```python
from build123d import *

# Parameters (mm, degrees)
BOSS_EXTRUDE1_DEPTH = 3
CUT_EXTRUDE3_DEPTH  = 4


with BuildPart() as part:
    # Sketch1 → Boss-Extrude1 (new body)
    with BuildSketch(Plane(origin=(0, 0, 0), x_dir=(1, 0, 0), z_dir=(0, 1, 0))):
        Polygon((-6, 15), (-9, 15), (-9, 0), (9, 0), (9, 15), (6, 15), (0, 9), align=None)
    extrude(amount=BOSS_EXTRUDE1_DEPTH)

    # Sketch6 → Cut-Extrude3 (cut, through all)
    with BuildSketch(Plane(origin=(0, 0, 0), x_dir=(1, 0, 0), z_dir=(0, 1, 0))):
        Polygon((-5.9, 3.1), (-5.9, 10.1), (-9.1, 10.1), (-9.1, -0.1), (-2.4, -0.1), (-2.4, 3.1), align=None)
        Polygon((9.1, 10.1), (5.9, 10.1), (5.9, 3.1), (2.4, 3.1), (2.4, -0.1), (9.1, -0.1), align=None)
    extrude(amount=CUT_EXTRUDE3_DEPTH, mode=Mode.SUBTRACT)


solid = part.part
```
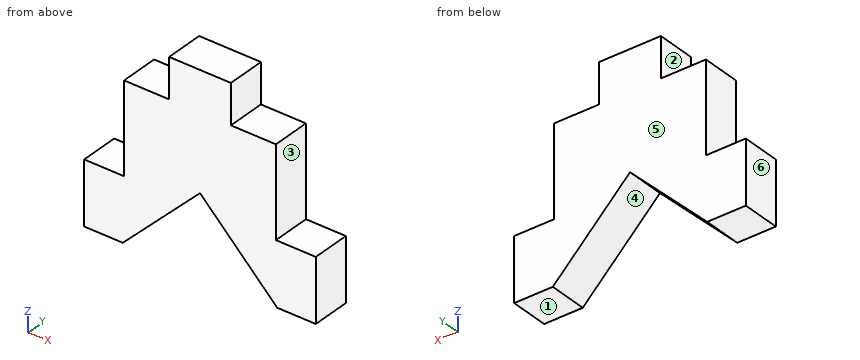
The listing builds one solid part. Answer for the finished solid, in the listing's coordinates (mm). Face numbers are marked on the shaded views. A direction names the side the tool comes from. Coordinates: 2 decimals unless noted, no trailing zeros. Write each loop counter-clockwise with the first axis right and the second up, starting at its lowest first coordinate (ties: lowest second). Pieces come first, ordered by that corner, then holes.
Q1. Given P1, Ø4, axis at x = -6.5, z = -13, coming from the -Y side; P2, Ø0.9, axis at y = 1.5, z = -5, coming from the -X side; P3, Ø0.9, axis at x = -3.5, y = 2, coming from the +Z side; P4, Ø0.9, axis at y = 1, z = -1, coming from the +X side, each flat-ended and moving along its own axis, determine where each tip first touches the part or whether it passes through.
Returned:
P1: stops at y = 0
P2: stops at x = -5.9
P3: stops at z = -3.1
P4: stops at x = 2.4
Q2. The mould has two halves that part along X. Classify the marked faces 4, 5 and 6: released by +X, released by -X, zero draft, split by the parting line, or undercut.
Returned:
face 4: undercut
face 5: zero draft
face 6: released by -X
Q3. Find the intervals of material crossed by line 1 along X through (y, z) = (2.2, -12.5); line 2 along X through (y, z) = (1.8, -10.5); line 3 along Z through (x, y) = (7.25, 1.1), in increasing order.
Returned:
line 1: x = -9 to -3.5, 3.5 to 9
line 2: x = -9 to -1.5, 1.5 to 9
line 3: z = -15 to -10.1
Q4. Section B-B, the plane y = 1.75 is taken. Write down the section's boundary in (x, z).
Returned:
outline: (-9, -15) - (-6, -15) - (0, -9) - (6, -15) - (9, -15) - (9, -10.1) - (5.9, -10.1) - (5.9, -3.1) - (2.4, -3.1) - (2.4, 0) - (-2.4, 0) - (-2.4, -3.1) - (-5.9, -3.1) - (-5.9, -10.1) - (-9, -10.1) - close
Q5. Which of the six approach directions +Z, -Z, +X, -X, +Y, -Y give full straight-line access (tool end or side, diameter ignored) to the marked faces 1, 2 and 3?
Returned:
face 1: -Z, +X, -X, +Y, -Y
face 2: +Z, -X, +Y, -Y
face 3: +Z, +X, +Y, -Y
Q6. Section C-C, the plane z = -14 is taken. Write down the section's boundary in (x, y), then the cut area to 3 significant figures.
Returned:
outline: (-9, 0) - (-5, 0) - (-5, 3) - (-9, 3) - close; (5, 0) - (9, 0) - (9, 3) - (5, 3) - close
area: 24.0 mm2
Q7. Section D-D, the plane x = -1.5 is taken. Write down the section's boundary in (y, z).
Returned:
outline: (0, -10.5) - (3, -10.5) - (3, 0) - (0, 0) - close
Q8. Section A-A, the plane z = -12.5 is taken. Write down the section's boundary in (x, y), then the cut area to 3 significant figures.
Returned:
outline: (-9, 0) - (-3.5, 0) - (-3.5, 3) - (-9, 3) - close; (3.5, 0) - (9, 0) - (9, 3) - (3.5, 3) - close
area: 33.0 mm2
